from build123d import *

# Parameters (mm, degrees)
BOSS_EXTRUDE1_DEPTH   = 50
BOSS_EXTRUDE1_2_DEPTH = 50
SKETCH1_3_R           = 15
BOSS_EXTRUDE2_DEPTH   = 20
BOSS_EXTRUDE3_DEPTH   = 19
SKETCH1_5_R           = 15
SKETCH1_5_R_2         = 11
BOSS_EXTRUDE4_DEPTH   = 13


with BuildPart() as part:
    # Sketch1 → Boss-Extrude1 (new body)
    with BuildSketch(Plane(origin=(0, 0, 0), x_dir=(1, 0, 0), z_dir=(0, 1, 0))):
        with BuildLine():
            Line((-33, 61), (-50, 61))
            Line((-50, 61), (-50, -23.561575886))
            ThreePointArc((-50, -23.561575886), (-41.631074926, -27.200063435), (-33, -30.163514831))
            Line((-33, -30.163514831), (-33, 61))
        make_face()
    extrude(amount=BOSS_EXTRUDE1_DEPTH)



with BuildPart() as body_2:
    # Sketch1 → Boss-Extrude1 2 (new body)
    with BuildSketch(Plane(origin=(0, 0, 0), x_dir=(1, 0, 0), z_dir=(0, 1, 0))):
        with BuildLine():
            Line((50, -23.561575886), (50, 61))
            Line((50, 61), (33, 61))
            Line((33, 61), (33, -30.163514831))
            ThreePointArc((33, -30.163514831), (41.631074926, -27.200063435), (50, -23.561575886))
        make_face()
    extrude(amount=BOSS_EXTRUDE1_2_DEPTH)


with BuildPart() as part_1:
    add(part.part)

    add(body_2.part)  # Boss-Extrude2 merges body 2
    # Sketch1_3 → Boss-Extrude2 (add)
    with BuildSketch(Plane(origin=(0, 0, 0), x_dir=(1, 0, 0), z_dir=(0, 1, 0))):
        with BuildLine():
            Line((33, 61), (-33, 61))
            Line((-33, 61), (-33, -30.163514831))
            ThreePointArc((-33, -30.163514831), (0, -35), (33, -30.163514831))
            Line((33, -30.163514831), (33, 61))
        make_face()
        with Locations(Location((0, 0, 0), (0, 0, 270))):
            Circle(SKETCH1_3_R, mode=Mode.SUBTRACT)
    extrude(amount=BOSS_EXTRUDE2_DEPTH)

    # Sketch1_4 → Boss-Extrude3 (add)
    with BuildSketch(Plane(origin=(0, 0, 0), x_dir=(1, 0, 0), z_dir=(0, 1, 0))):
        with BuildLine():
            ThreePointArc((50, 103.561575886), (0, 115), (-50, 103.561575886))
            Line((-50, 103.561575886), (-50, 61))
            Line((-50, 61), (-33, 61))
            Line((-33, 61), (33, 61))
            Line((33, 61), (50, 61))
            Line((50, 61), (50, 103.561575886))
        make_face()
        with BuildLine():
            ThreePointArc((-30.545454545, 91.010852136), (0, 96), (30.545454545, 91.010852136))
            ThreePointArc((30.545454545, 91.010852136), (35.584237678, 80.881159913), (25.454545455, 75.84237678))
            ThreePointArc((25.454545455, 75.84237678), (0, 80), (-25.454545455, 75.84237678))
            ThreePointArc((-25.454545455, 75.84237678), (-35.584237678, 80.881159913), (-30.545454545, 91.010852136))
        make_face(mode=Mode.SUBTRACT)
    extrude(amount=BOSS_EXTRUDE3_DEPTH)

    # Sketch1_5 → Boss-Extrude4 (add)
    with BuildSketch(Plane(origin=(0, 0, 0), x_dir=(1, 0, 0), z_dir=(0, 1, 0))):
        with Locations(Location((0, 0, 0), (0, 0, 270))):
            Circle(SKETCH1_5_R)
        with Locations(Location((0, 0, 0), (0, 0, 90))):
            Circle(SKETCH1_5_R_2, mode=Mode.SUBTRACT)
    extrude(amount=BOSS_EXTRUDE4_DEPTH)

    # Sketch3 → Cut-Revolve1 (revolve, cut)
    with BuildSketch(Plane(origin=(0, 35, 0), x_dir=(1, 0, 0), z_dir=(0, 1, 0))):
        Polygon((-50, 53.34), (50, 54), (50, 47), (-50, 47), align=None)
    revolve(axis=Axis((-50, 35, -47), (1, 0, 0)), mode=Mode.SUBTRACT)


solid = part_1.part
Read the model definition and answer for the solid it produces. Units are mm, in the model's axes. A direction names the side the tool comes from. Round coordinates to 2 decimals unless told otherwise and drop trailing zeros. Order: outer loops, then holes, each group sorted by start corner. A loop starts at its lowest first (then second) coordinate and runs counter-clockwise, first axis right, second up. Notation, with made-up numbers: (11.5, 22.5) - (58.5, 22.5) arc R27 cw to (58.5, 42.5) - close; hole circle Ø11 at (47.5, -32). An arc over 180 degrees is marked (long way). Use one line per item in the form item = value. Start each with the question number.
(1) The part is cut by section C-C (z = 0). Give the vertices of the cut face in (x, y), then the cut area to 3 significant figures.
(2) A flat-ended cylindrical pin translates along its axis: pin 1 Ø5 at (x, z) = (-21, -29) entering from +Y. Find the tip coordinate at first contact, or state that the pin passes through.
(3) The part is cut by section B-B (x = 0). Give the vertices of the cut face in (y, z), then the cut area to 3 significant figures.
(4) For faces 4 (the face through (-33, 35, -15)), 5 (the face through (-3.5, 19.5, -61)), 6 (the face through (41.6, 32.3, -53.4)), determine the directions among +Z, -Z, +X, -X, +Y, -Y from which every point of the face is accessible in a straight line to the end or side of a thin tool.
(5) The part is cut by section A-A (y = 7.5). Give the vertices of the cut face in (x, z), then the cut area to 3 significant figures.
(6) The part is cut by section D-D (y = 21.5). Give the vertices of the cut face in (x, z).
(7) Determine the mould class of faces 1 (the face through (-41.38, 36.92, -53.1)), 2 (the face through (10, 13, -5)), 3 (the face through (0, 9, -96)) for opening direction Y: +Y half, -Y half, draft (parallel to the pull), parting line (faces both ways), or undercut.
(8) Find the intervals of material crossed by line 1 along X through (y, z) = (34, 6.5); line 2 along Z through (x, y) = (13.5, 16); line 3 along X through (y, z) = (2.5, 0), in increasing order. Write a range as from..to.
Checked values:
q1.outline = (-50, 0) - (-11, 0) - (-11, 13) - (-15, 13) - (-15, 20) - (-33, 20) - (-33, 50) - (-50, 50) - close; (11, 0) - (50, 0) - (50, 50) - (33, 50) - (33, 20) - (15, 20) - (15, 13) - (11, 13) - close
q1.area = 2,520 mm^2
q2.pin_1 = 20
q3.outline = (0, -115) - (19, -115) - (19, -96) - (0, -96) - close; (0, -80) - (19, -80) - (19, -61) - (20, -61) - (20, -15) - (13, -15) - (13, -11) - (0, -11) - close; (0, 11) - (13, 11) - (13, 15) - (20, 15) - (20, 35) - (0, 35) - close
q3.area = 2,150 mm^2
q4.face_4 = +Z, -Z, +Y
q4.face_5 = -Z, +X, -X, +Y
q4.face_6 = +X
q5.outline = (-50, -103.56) arc R115 ccw to (50, -103.56) - (50, 23.56) arc R115 ccw to (-50, 23.56) - close; hole (-30.55, -91.01) arc R96 ccw to (30.55, -91.01) arc R8 ccw to (25.45, -75.84) arc R80 cw to (-25.45, -75.84) arc R8 ccw to start; hole circle Ø22 at (0, 0)
q5.area = 12,800 mm^2
q6.outline = (-50, -61) - (-33, -61) - (-33, 30.16) arc R115 ccw to (-50, 23.56) - close; (33, -61) - (50, -61) - (50, 23.56) arc R115 ccw to (33, 30.16) - close
q7.face_1 = undercut
q7.face_2 = +Y half
q7.face_3 = draft
q8.line_1 = -50..-33, 33..50
q8.line_2 = -114.2..-95.05, -78.85..-6.54, 6.54..34.2
q8.line_3 = -50..-11, 11..50
